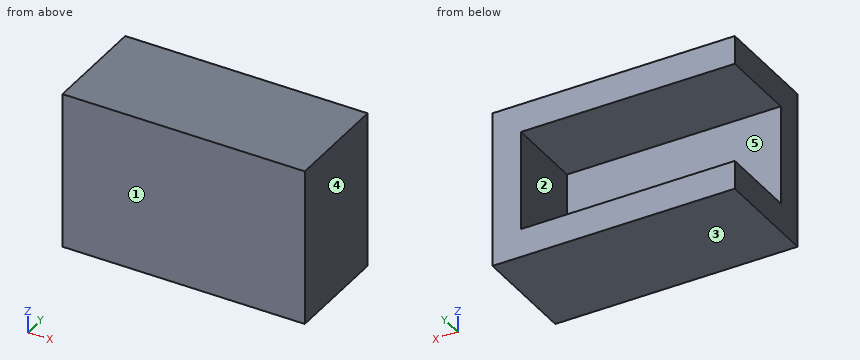
Autodesk Inventor part; units mm, degrees
ref_plane "YZ Plane" through (0, 0, 0) normal (1, 0, 0) x (0, 1, 0)
ref_plane "XZ Plane" through (0, 0, 0) normal (0, 1, 0) x (-1, 0, 0)
ref_plane "XY Plane" through (0, 0, 0) normal (0, 0, 1) x (1, 0, 0)
sketch "Sketch1" plane through (0, 0, 0) normal (0, 1, 0) x (-1, 0, 0)
  line L0 (-15, 7) -> (-15, -7)
  line L1 (-15, -7) -> (15, -7)
  line L2 (15, -7) -> (15, 7)
  line L3 (15, 7) -> (-15, 7)
  line L4 (-15, 7) -> (15, -7) construction
  line L5 (-15, -7) -> (15, 7) construction
  line L6 (-19, 11) -> (-19, -11)
  line L7 (-19, -11) -> (19, -11)
  line L8 (19, -11) -> (19, 11)
  line L9 (19, 11) -> (-19, 11)
  line L10 (15, 7) -> (15, 11)
  line L11 (15, -7) -> (15, -11)
  point P0 (0, 0)
  dimension "d0" = 14
  dimension "d1" = 30
  dimension "d2" = 4
extrude "Extrusion1" add sketch "Sketch1" along normal blind 15 contours L0 L1 L11 L7 L6 L9 L10 L3
extrude "Extrusion2" add sketch "Sketch1" along normal blind 4 contours L3 L2 L1 L0
properties part number "Solenoid Mount"
Can you work these out from the model? Positions are in its coordinate system, mm. Face numbers are marked on the shaded views. A direction names the side the tool comes from. Give positions to 0.01 mm unless a question says otherwise; leave off trailing zeros. Write each loop counter-clockwise with the first axis right and the second up, starting at its lowest first coordinate (ties: lowest second). Pieces come first, ordered by that corner, then holes. Notation, with made-up numbers: M 32.25,27.5 L 68.25,27.5 A20 cw 68.25,58.5 Z; hole C 37,22.5 d1. An arc over 180 degrees is marked long. Answer in a Markdown table with one row per item. Add a question column.
Item 1: We'd pull the mould along Z, two halves only. Please class the marked faces 1, 2 and 3: released by +Z, released by -Z, zero draft, split by the parting line, or undercut.
Item 2: On a 3-axis mill with a long thin cutter (end or side, diameter ignored), from which of +Z, -Z, +X, -X, +Y, -Y can I reach the whole of each face in a straight line? I mean the marked faces 4 and 5. Say none if no direction works.
Item 3: Please list where these lines run through material, in increasing order: L1, parallel to Z at x = 8, y = 9.25; L2, parallel to X at y = 10, z = 2.5; L3, parallel to Y at x = 0.5, z = 3.
Item 4: Imagine slicing it at A-A, the plane z = -2.5. Write out the boundary of the cut face in (x, y), plus the area to 3 significant figures.
Item 5: Imagine slicing it at B-B, the plane y = 14. Write out the boundary of the cut face in (x, z).
Item 6: Imagine slicing it at C-C, the plane x = -8. Write out the boundary of the cut face in (y, z).
Item 7: For pin 1 Ø12 at (x, z) = (-2.5, -2) entering from -Y, with a flat end and sliding along its axis, tell me the tip position at first contact or that it passes through.
Evaluation:
| question | item | result |
|---|---|---|
| 1 | face 1 | zero draft |
| 1 | face 2 | undercut |
| 1 | face 3 | released by -Z |
| 2 | face 4 | +Z, -Z, +X, +Y, -Y |
| 2 | face 5 | -X, +Y |
| 3 | L1 | z = -11 to -7, 7 to 11 |
| 3 | L2 | x = 15 to 19 |
| 3 | L3 | y = 0 to 4 |
| 4 | outline | M -15,0 L 19,0 L 19,15 L 15,15 L 15,4 L -15,4 Z |
| 4 | area | 180 mm² |
| 5 | outline | M -15,-11 L 19,-11 L 19,11 L -15,11 L -15,7 L 15,7 L 15,-7 L -15,-7 Z |
| 6 | outline | M 0,-11 L 15,-11 L 15,-7 L 4,-7 L 4,7 L 15,7 L 15,11 L 0,11 Z |
| 7 | pin 1 | stops at y = 0 |
